```python
from build123d import *

# Parameters (mm, degrees)
SKETCH2_OUTSIDE_W       = 10.368
SKETCH2_OUTSIDE_H       = 10.368
SKETCH2_OUTSIDE_R       = 2.8
CUT_EXTRUDE1_DEPTH      = 10.06513549
FILLET1_R               = 0.8
ENL_V_MAT_EXTRU_1_DEPTH = 1


with BuildPart() as part:
    # Sketch1 → Base-Revolve (revolve)
    with BuildSketch(Plane(origin=(0, 0, 0), x_dir=(0, 0, -1), z_dir=(1, 0, 0))):
        Polygon((1.65, 0), (1.65, 3.0146875), (0, 1.3646875), (-0.765631875, 1.3646875), (-1, 1.5), (-6.35, 1.5), (-6.35, 0), align=None)
    revolve(axis=Axis((0, 0, -1.65), (0, 0, 1)))

    # Sketch2 outside → Cut-Extrude1 (cut, through all)
    with BuildSketch(Plane(origin=(0, 0, -1.65), x_dir=(-1, 0, 0), z_dir=(0, 0, -1))):
        Rectangle(SKETCH2_OUTSIDE_W, SKETCH2_OUTSIDE_H)
        with Locations(Location((0, 0, 0), (0, 0, 90))):
            Circle(SKETCH2_OUTSIDE_R, mode=Mode.SUBTRACT)
    extrude(amount=-CUT_EXTRUDE1_DEPTH, mode=Mode.SUBTRACT)

    # Fillet1
    fillet1_edges = [part.edges().sort_by_distance(p)[0] for p in [
        (0, -1.3646875, 0),
    ]]
    fillet(fillet1_edges, radius=FILLET1_R)

    # Esquisse1 → Enlèv. mat.-Extru.1 (cut)
    with BuildSketch(Plane(origin=(0, 0, -1.65), x_dir=(-1, 0, 0), z_dir=(0, 0, -1))):
        with BuildLine():
            ThreePointArc((1.088832331, -0.880025088), (1.212435565, -0.7), (1.306540248, -0.502943915))
            ThreePointArc((1.306540248, -0.502943915), (1.025, 0), (1.306540248, 0.502943915))
            ThreePointArc((1.306540248, 0.502943915), (1.212435565, 0.7), (1.088832331, 0.880025088))
            ThreePointArc((1.088832331, 0.880025088), (0.5125, 0.887676039), (0.217707917, 1.382969003))
            ThreePointArc((0.217707917, 1.382969003), (0, 1.4), (-0.217707917, 1.382969003))
            ThreePointArc((-0.217707917, 1.382969003), (-0.5125, 0.887676039), (-1.088832331, 0.880025088))
            ThreePointArc((-1.088832331, 0.880025088), (-1.212435565, 0.7), (-1.306540248, 0.502943915))
            ThreePointArc((-1.306540248, 0.502943915), (-1.025, 0), (-1.306540248, -0.502943915))
            ThreePointArc((-1.306540248, -0.502943915), (-1.212435565, -0.7), (-1.088832331, -0.880025088))
            ThreePointArc((-1.088832331, -0.880025088), (-0.5125, -0.887676039), (-0.217707917, -1.382969003))
            ThreePointArc((-0.217707917, -1.382969003), (0, -1.4), (0.217707917, -1.382969003))
            ThreePointArc((0.217707917, -1.382969003), (0.5125, -0.887676039), (1.088832331, -0.880025088))
        make_face()
    extrude(amount=-ENL_V_MAT_EXTRU_1_DEPTH, mode=Mode.SUBTRACT)


solid = part.part
```
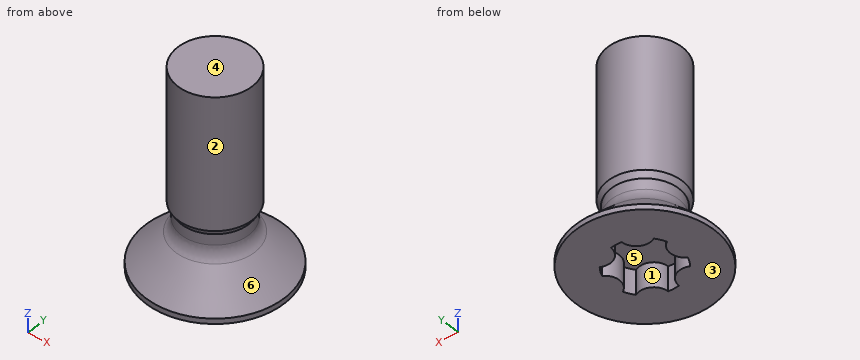
Check sheet for the modelled part. Datum: model origin and axes. Units: mm. Face numbers are marked on the shaded views. A direction names the side the tool comes from. Coordinates: 2 decimals unless noted, no trailing zeros. Order: outer loops, then holes, each group sorted by start corner. A loop starts at its lowest first (then second) coordinate and runs counter-clockwise, first axis right, second up. Notation, with made-up numbers: (14, 43.5) -> (30, 43.5) arc R10 cw to (30, 57.5) -> close; hole circle Ø5 at (-34.5, 76). An arc over 180 degrees is marked (long way). Write item = value, one per line. Start each with the question number.
1) Material ranges on L1, parallel to Z at x = 0.15, y = 0; L2, parallel to Y at x = -0.05, z = 4.75; L3, parallel to Z at x = -2.55, y = 0.3, recorded low to high.
2) Mould release check, pull along Y, two halves, no side actions. Record for the marked faces 4, 5 and 6: +Y half, -Y half, draft (parallel to the pull), parting line (faces both ways), or undercut.
3) Cross-section at B-B (z = 0.5). Enter the section's corners in (x, y).
4) Cross-section at A-A (z = 4.5). Enter the section's corners in (x, y).
5) Access from +Z, -Z, +X, -X, +Y, -Y to the whole of each face (thin tool, end or side, straight path). Record for the marked faces 1, 2 and 3.
6) Go/stop test with flat-tipped pins: P1, Ø1, axis at y = 1.5, z = 2.5, coming from the -X side; P2, Ø1.3, axis at x = 0, y = -0.5, coming from the -Z side; P3, Ø1.5, axis at x = 1, z = 0, coming from the -Y side. Record where each tip stops, or that it passes through.
Ans:
q1.L1 = -0.65 to 6.35
q1.L2 = -1.5 to 1.5
q1.L3 = -1.65 to -1.2
q2.face_4 = draft
q2.face_5 = undercut
q2.face_6 = parting line
q3.outline = circle Ø2.73 at (0, 0)
q4.outline = circle Ø3 at (0, 0)
q5.face_1 = -Z
q5.face_2 = +Z
q5.face_3 = -Z, +X, -X, +Y, -Y
q6.P1 = -1.12
q6.P2 = -1.65
q6.P3 = -1.93
